The model under review builds one solid part; all positions refer to its coordinate system, in mm. Give positions to 0.01 mm unless a question says otherwise; leave off trailing zeros. Write each loop counter-clockwise with the first axis right and the second up, starting at its lowest first coordinate (ties: lowest second). Pieces come first, ordered by that corner, then holes. Notation, with made-up numbers: (36.5, -31.75) - (89.5, -31.75) arc R12 ccw to (89.5, -12.75) - close; hole circle Ø2 at (39, 4.5). An arc over 180 degrees is marked (long way). Write item = value, one per line.
```python
from build123d import *

# Parameters (mm, degrees)
SKETCH1_W           = 120
SKETCH1_H           = 120
BOSS_EXTRUDE1_DEPTH = 4
FILLET1_R           = 19


with BuildPart() as part:
    # Sketch1 → Boss-Extrude1 (new body)
    with BuildSketch(Plane(origin=(0, 0, 0), x_dir=(1, 0, 0), z_dir=(0, 1, 0))):
        with Locations((60, 60)):
            Rectangle(SKETCH1_W, SKETCH1_H)
    extrude(amount=BOSS_EXTRUDE1_DEPTH)

    # Fillet1
    fillet1_edges = [part.edges().sort_by_distance(p)[0] for p in [
        (0, 2, -120),
        (120, 2, -120),
        (120, 2, 0),
        (0, 2, 0),
    ]]
    fillet(fillet1_edges, radius=FILLET1_R)


solid = part.part
```
1. Take a section at B-B on x = 110. Give the boundary of the cut face in (y, z), and give its area (3 significant figures).
Findings below:
outline = (0, -117.73) - (4, -117.73) - (4, -2.27) - (0, -2.27) - close
area = 462 mm²
2. For line 1 (X direction, y = 0.25, z = -113.5); line 2 (Z direction, x = 104.5, y = 0.55); line 3 (X direction, y = 2.1, z = -14.5), list the stretches that pass through material, from the lowest coordinate up. Write a range as from..to.
Findings below:
line_1 = 4.69..115.31
line_2 = -119.67..-0.33
line_3 = 0.54..119.46
3. Take a section at A-A on y = 2.25. Give the boundary of the cut face in (x, z), and give its area (3 significant figures).
Findings below:
outline = (0, -101) arc R19 ccw to (19, -120) - (101, -120) arc R19 ccw to (120, -101) - (120, -19) arc R19 ccw to (101, 0) - (19, 0) arc R19 ccw to (0, -19) - close
area = 14,100 mm²
